Geometry: final body of the model. Coordinates: model frame, mm. A direction names the side the tool comes from. Coordinates: 2 decimals unless noted, no trailing zeros. Write each loop counter-clockwise with the first axis right and the second up, starting at its lowest first coordinate (ties: lowest second). Pieces come first, ordered by that corner, then holes. Notation, with made-up numbers: M 46.25,71 L 83.25,71 A27 ccw 83.25,91 Z; hole C -15,59.5 d5. An arc over 180 degrees is marked long. Write item = value, one per line. Start each with the question number.
Item 1: Pull-direction query (X, two-part tool) for faces 1 (the flat face through (-13, -2.725, 6)), 2 (the flat face through (12.006, 23, 6)), 3 (the flat face through (-9.261, -12, 6)), 4 (the flat face through (-14, -12, 6)); classes: +X half, -X half, draft (parallel to the pull), parting line (faces both ways), or undercut.
Item 2: Section D-D on y = 8.5. Output: boundary loops of the cut face in (x, z), plus the area to 3 significant figures.
Item 3: Reachability of faces 5 (the flat face through (-11.994, 23, 6)), 6 (the flat face through (0, 20, 0)), 7 (the flat face through (0, 20, 12)), 8 (the flat face through (9.261, -12, 6)), 9 (the flat face through (13, -2.727, 6)) from +Z, -Z, +X, -X, +Y, -Y: full face, straight path, thin tool, end or side. Return the list, or none.
Item 4: Section B-B on x = -0.25. Output: boundary loops of the cut face in (y, z).
Item 5: Ray query, L1, parallel to Y at x = -7, z = 3; L2, parallel to X at y = -14, z = 1.25; L3, parallel to X at y = 7.5, z = 3.5. Return the intervals inside material, ascending. Write a range as [from, to].
Item 6: Section C-C on z = 7.5. Output: boundary loops of the cut face in (x, y).
Item 7: First-contact query: pin 1 Ø5 at (y, z) = (44.77, 3) entering from +X; pin 2 Ø3 at (x, z) = (0.5, 8) entering from +Y; pin 3 Ø1 at (x, z) = (13, 6.5) entering from +Y. Flat tips, straight axial feed; report the tip coordinate or a pass-through.
Item 8: Section A-A on z = 3. Output: boundary loops of the cut face in (x, y).
from build123d import *

# Parameters (mm, degrees)
EXTRUDE_1_DEPTH      = 12
EXTRUDE_4_DEPTH      = 24
SKETCH_16_R          = 2
CUT_EXTRUDE_11_DEPTH = 27.005399728


with BuildPart() as part:
    # 스케치1 → 보스-돌출1 (new body)
    with BuildSketch(Plane.XY):
        Polygon((-11.994395335, 44.774969809), (-11.994395335, -2.725030191), (-13.999795062, -2.725030191), (-13.999795062, -20.993190191), (-9.261084312, -20.993190191), (-9.261084312, -2.725030191), (9.261494188, -2.727088258), (9.261494188, -20.993190191), (14.000204938, -20.993190191), (14.000204938, -2.727088258), (12.005604665, -2.727088258), (12.005604665, 44.774969809), align=None)
    extrude(amount=EXTRUDE_1_DEPTH)

    # 스케치15 → 보스-돌출4 (add)
    with BuildSketch(Plane(origin=(12.005604665, 0, 0), x_dir=(0, 0, -1), z_dir=(1, 0, 0))):
        with BuildLine():
            Line((-12, 44.774969809), (-3.746682541, 47.680561863))
            ThreePointArc((-3.746682541, 47.680561863), (-1.161528845, 47.145628749), (0, 44.774969809))
            Line((0, 44.774969809), (-12, 44.774969809))
        make_face()
    extrude(amount=-EXTRUDE_4_DEPTH)

    # 스케치16 → 컷-돌출11 (cut, through all)
    with BuildSketch(Plane(origin=(12.005604665, 0, 0), x_dir=(0, 0, -1), z_dir=(1, 0, 0))):
        with Locations((-3, 44.774969809)):
            Circle(SKETCH_16_R)
    extrude(amount=-CUT_EXTRUDE_11_DEPTH, mode=Mode.SUBTRACT)


solid = part.part
Responses:
q1.face_1 = draft
q1.face_2 = +X half
q1.face_3 = undercut
q1.face_4 = -X half
q2.outline = M -11.99,0 L 12.01,0 L 12.01,12 L -11.99,12 Z
q2.area = 288 mm²
q3.face_5 = +Z, -Z, -X, +Y
q3.face_6 = -Z, +X, -X, +Y, -Y
q3.face_7 = +Z, +X, -X, +Y, -Y
q3.face_8 = +Z, -Z, -Y
q3.face_9 = +Z, -Z, +X, +Y
q4.outline = M -2.73,0 L 44.77,0 A3 ccw 47.68,3.75 L 44.77,12 L -2.73,12 Z; hole C 44.77,3 d4
q5.L1 = [-2.73, 42.77], [46.77, 47.77]
q5.L2 = [-14, -9.26], [9.26, 14]
q5.L3 = [-11.99, 12.01]
q6.outline = M -14,-20.99 L -9.26,-20.99 L -9.26,-2.73 L 9.26,-2.73 L 9.26,-20.99 L 14,-20.99 L 14,-2.73 L 12.01,-2.73 L 12.01,46.36 L -11.99,46.36 L -11.99,-2.73 L -14,-2.73 Z
q7.pin_1 = 12.01
q7.pin_2 = 46.71
q7.pin_3 = -2.73
q8.outline = M -14,-20.99 L -9.26,-20.99 L -9.26,-2.73 L 9.26,-2.73 L 9.26,-20.99 L 14,-20.99 L 14,-2.73 L 12.01,-2.73 L 12.01,42.77 L -11.99,42.77 L -11.99,-2.73 L -14,-2.73 Z; M -11.99,46.77 L 12.01,46.77 L 12.01,47.77 L -11.99,47.77 Z
